Geometry check sheet. Reference: drawing and pictorial views, mm from the part's lowest x, y, z. A direction names the side the tool comes from. Coordinates: 2 decimals unless noted, no trailing zeros. Write each loop counter-clockwise with the first axis right and the second up, starting at its lowest first coordinate (ties: lowest second). Pieces come first, ordered by that corner, then holes. Notation, with made-up numbers: (41.5, 20.5) -> (46.5, 20.5) arc R31 cw to (46.5, 54.5) -> close; hole circle Ø2 at (21.25, 27.5). An arc over 180 degrees is marked (long way). Answer in a Markdown table with one row per item.
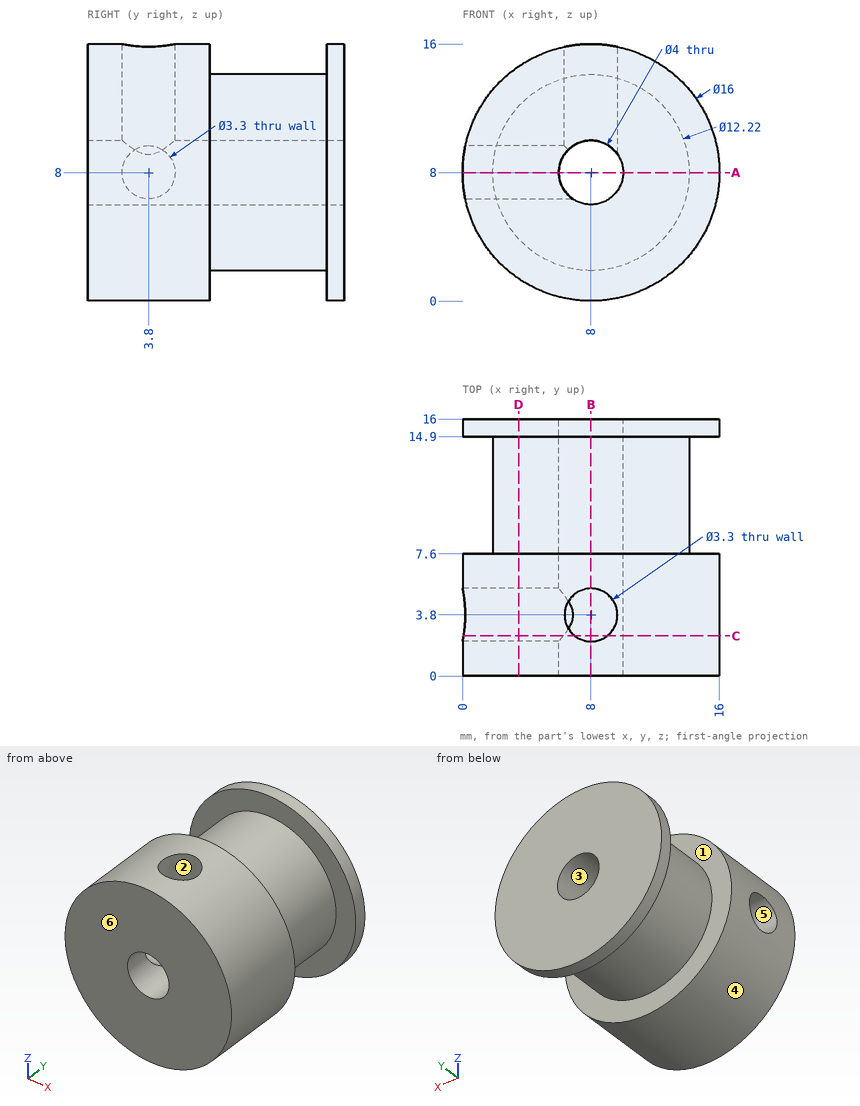
1. Tool access check on the marked faces 1, 2 and 3. Record the directions out of +Z, -Z, +X, -X, +Y, -Y that give a thin tool (end or side, any length) a straight path to the whole face; none if there is none.
Geometry says:
| item | result |
|---|---|
| face 1 | none |
| face 2 | +Z |
| face 3 | +Y, -Y |
2. Thickness scan on line 1 (Y direction, x = 11.75, z = 2.75); line 2 (X direction, y = 6, z = 8); line 3 (Z direction, x = 9.25, y = 14.25). Record the ranges inside material, lowest first. Write a range as from..to.
Geometry says:
| item | result |
|---|---|
| line 1 | 0..7.6, 14.9..16 |
| line 2 | 0..6, 10..16 |
| line 3 | 2.02..6.44, 9.56..13.98 |
3. Section check B-B, the plane x = 8. Record the boundary of the cut face in (y, z).
Geometry says:
| item | result |
|---|---|
| outline | (0, 0) -> (7.6, 0) -> (7.6, 1.89) -> (14.9, 1.89) -> (14.9, 0) -> (16, 0) -> (16, 6) -> (0, 6) -> close; (0, 10) -> (2.15, 10) -> (2.15, 16) -> (0, 16) -> close; (5.45, 10) -> (16, 10) -> (16, 16) -> (14.9, 16) -> (14.9, 14.11) -> (7.6, 14.11) -> (7.6, 16) -> (5.45, 16) -> close |
4. Section check C-C, the plane y = 2.5. Record the boundary of the cut face in (x, z), plus the area to 3 significant figures.
Geometry says:
| item | result |
|---|---|
| outline | (0.06, 6.98) arc R8 ccw (long way) to (9.02, 15.94) -> (9.02, 9.72) arc R2 cw (long way) to (6.28, 6.98) -> close; (0.06, 9.02) -> (6.28, 9.02) arc R2 cw to (6.98, 9.72) -> (6.98, 15.94) arc R8 ccw to start |
| area | 164 mm^2 |
5. Depth check by flat-ended pin: P1, Ø2, axis at y = 4.5, z = 6, coming from the +X side; P2, Ø5, axis at y = 10.5, z = 14, coming from the +X side; P3, Ø6, axis at y = 11.5, z = 12.5, coming from the +X side; P4, Ø4, axis at x = 8, y = 3.8, coming from the +Z side. Enter the tip coordinate at first touch or a pass-through.
Geometry says:
| item | result |
|---|---|
| P1 | x = 15.94 |
| P2 | x = 13.01 |
| P3 | x = 13.92 |
| P4 | z = 16 |
6. Section check D-D, the plane x = 3.5. Record the boundary of the cut face in (y, z), plus the area to 3 significant figures.
Geometry says:
| item | result |
|---|---|
| outline | (0, 1.39) -> (7.6, 1.39) -> (7.6, 3.87) -> (14.9, 3.87) -> (14.9, 1.39) -> (16, 1.39) -> (16, 14.61) -> (14.9, 14.61) -> (14.9, 12.13) -> (7.6, 12.13) -> (7.6, 14.61) -> (0, 14.61) -> close; hole circle Ø3.3 at (3.8, 8) |
| area | 167 mm^2 |
7. Mould release check, pull along Z, two halves, no side actions. Record for the marked faces 4, 5 and 6: released by +Z, released by -Z, zero draft, split by the parting line, or undercut.
Geometry says:
| item | result |
|---|---|
| face 4 | split by the parting line |
| face 5 | undercut |
| face 6 | zero draft |
8. Section check A-A, the plane z = 8. Record the boundary of the cut face in (x, y).
Geometry says:
| item | result |
|---|---|
| outline | (0, 0) -> (6, 0) -> (6, 2.15) -> (0, 2.15) -> close; (0, 5.45) -> (6, 5.45) -> (6, 16) -> (0, 16) -> (0, 14.9) -> (1.89, 14.9) -> (1.89, 7.6) -> (0, 7.6) -> close; (10, 0) -> (16, 0) -> (16, 7.6) -> (14.11, 7.6) -> (14.11, 14.9) -> (16, 14.9) -> (16, 16) -> (10, 16) -> close |
